Source: CAD feature listing. Evaluate the final solid. Frame: model axes, mm. Face numbers are marked on the shaded views. A direction names the side the tool comes from. Coordinates: 2 decimals unless noted, no trailing zeros. Loops run counter-clockwise (first coordinate to the right, second up) from the corner with the lowest first, then second, coordinate; pieces in that order, holes last. Notation, with made-up numbers: M 49,-11 L 53,-11 A23 ccw 53,9 Z; hole C 79.5,60.5 d9. An arc over 180 degrees is marked long. Write each question's results on one line, items separated by ' | '. Start each with the question number.
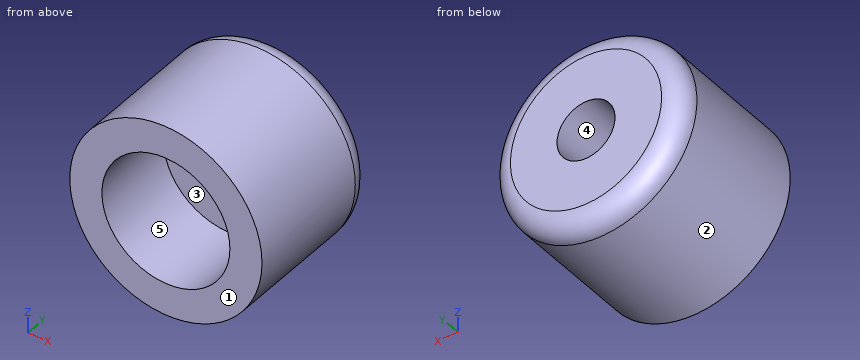
from build123d import *

# Parameters (mm, degrees)
F0_R     = 7.1501
F1_DEPTH = 11.1252
F2_R     = 2.159
F3_DEPTH = 11.1262
F4_R     = 4.7625
F5_DEPTH = 6.35
F6_R     = 1.524


with BuildPart() as f1:
    # F0 (on Front) → F1 (new body)
    with BuildSketch(Plane.XZ):
        Circle(F0_R)
    extrude(amount=F1_DEPTH)

    # F2 (on face) → F3 (cut, through all)
    with BuildSketch(Plane.XZ.offset(11.1252)):
        Circle(F2_R)
    extrude(amount=-F3_DEPTH, mode=Mode.SUBTRACT)

    # F4 (on face) → F5 (cut)
    with BuildSketch(Plane.XZ.offset(11.1252)):
        Circle(F4_R)
    extrude(amount=-F5_DEPTH, mode=Mode.SUBTRACT)

    # F6
    f6_edges = [f1.edges().sort_by_distance(p)[0] for p in [
        (-7.1501, 0, 0),
    ]]
    fillet(f6_edges, radius=F6_R)


solid = f1.part
Item 1: Cut plane C-C (y = -3.5). Output: boundary loops of the cut face in (x, z).
Item 2: Line query: probe 1 along Z at (x, y) = (0, -1.9); probe 2 along Z at (x, y) = (0, -8.5); probe 3 along Y at (x, z) = (1.25, -3.25). Output: solid intervals per line, ascending.
Item 3: Cut plane B-B (z = 0). Output: boundary loops of the cut face in (x, y).
Item 4: Access query for the marked faces 4 and 5. Directions: +Z, -Z, +X, -X, +Y, -Y. A direction counts if a zero-diameter tool reaches every point of the face in a straight line with its end or side. Return the directions, or none.
Item 5: Cut plane D-D (y = -5.25). Output: boundary loops of the cut face in (x, z) (1 decimal).
Item 6: Mould query, pull axis Z, two halves, no side actions, for the marked faces 1, 2 and 3. Classes: +Z half, -Z half, draft (parallel to the pull), parting line (faces both ways), or undercut.
Item 7: First-contact query: pin 1 Ø1 at (x, y) = (-1, -8) entering from -Z; pin 2 Ø3 at (x, y) = (3, -5.5) entering from -Z; pin 3 Ø6 at (y, z) = (-6.5, -4) entering from -X. Flat tips, straight axial feed; report the tip coordinate or a pass-through.
Item 8: Cut plane A-A (x = 0). Output: boundary loops of the cut face in (y, z), then the cut area to 3 significant figures.
Response values:
1) outline: C 0,0 d14.3; hole C 0,0 d4.32
2) probe 1: z = -7.15 to -2.16, 2.16 to 7.15 | probe 2: z = -7.15 to -4.76, 4.76 to 7.15 | probe 3: y = -4.78 to 0
3) outline: M -7.15,-11.13 L -4.76,-11.13 L -4.76,-4.78 L -2.16,-4.78 L -2.16,0 L -5.63,0 A1.52 ccw -7.15,-1.52 Z; M 2.16,-4.78 L 4.76,-4.78 L 4.76,-11.13 L 7.15,-11.13 L 7.15,-1.52 A1.52 ccw 5.63,0 L 2.16,0 Z
4) face 4: +Y, -Y | face 5: -Y
5) outline: C 0,0 d14.3; hole C 0,0 d9.5
6) face 1: draft | face 2: parting line | face 3: undercut
7) pin 1: stops at z = -7.13 | pin 2: stops at z = -6.99 | pin 3: stops at x = -7.08
8) outline: M -11.13,-7.15 L -1.52,-7.15 A1.52 ccw 0,-5.63 L 0,-2.16 L -4.78,-2.16 L -4.78,-4.76 L -11.13,-4.76 Z; M -11.13,4.76 L -4.78,4.76 L -4.78,2.16 L 0,2.16 L 0,5.63 A1.52 ccw -1.52,7.15 L -11.13,7.15 Z | area: 77.0 mm2
